from build123d import *

# Parameters (mm, degrees)
SKIZZE1_R                       = 9.5
AUFSATZ_LINEAR_AUSTRAGEN2_DEPTH = 12
SKIZZE9_R                       = 11
SCHNITT_LINEAR_AUSTRAGEN2_DEPTH = 10


with BuildPart() as part:
    # Skizze1 → Aufsatz-Linear austragen2 (new body)
    with BuildSketch(Plane.XY):
        Polygon((15, 15), (-15, 15), (-15, -40), (-5, -40), (-5, -20), (15, -20), align=None)
        Circle(SKIZZE1_R, mode=Mode.SUBTRACT)
    extrude(amount=AUFSATZ_LINEAR_AUSTRAGEN2_DEPTH)

    # Skizze9 → Schnitt-Linear austragen2 (cut)
    with BuildSketch(Plane(origin=(0, 0, 0), x_dir=(-1, 0, 0), z_dir=(0, 0, -1))):
        Circle(SKIZZE9_R)
    extrude(amount=-SCHNITT_LINEAR_AUSTRAGEN2_DEPTH, mode=Mode.SUBTRACT)


solid = part.part
Could you check a few things on this model? Use its own coordinates, in mm. A direction names the side the tool comes from. Give positions to 0.01 mm unless a question says otherwise; leave off trailing zeros. Write each loop counter-clockwise with the first axis right and the second up, starting at its lowest first coordinate (ties: lowest second). Pieces come first, ordered by that corner, then holes. Notation, with made-up numbers: (76.25, 13.5) - (102.25, 13.5) arc R24 ccw to (102.25, 27.5) - close; hole circle Ø3 at (62, 24.5). An arc over 180 degrees is marked (long way). Use CSV: the item, a comma, the result in double quotes. Start each with the question number.
Item 1: I want a section at B-B, the plane y = 0. Please give me the cut outline in (x, z), then the cut area to 3 significant figures.
Item 2: I'm going to push a flat-ended pin straight in: pin 1 (3.5 mm diameter, centred on x = 9.5, z = 8.5, fed in from -Y). Where does the tip first touch, or does it pass through?
Item 3: If I drill on line 1 along X through (y, z) = (0, 11.1); line 2 along Y through (x, z) = (0, 10.6); line 3 along X through (y, z) = (-25, 11.75), over which ranges is the centre line in solid material (lowest first)?
Item 4: I want a section at C-C, the plane z = 2.75. Please give me the cut outline in (x, y).
Item 5: For faces 4 (the face through (-10, -40, 6)), 5 (the face through (2.38, -10.74, 4.93)), 6 (the face through (-5, -30, 6)), which set-ups out of +Z, -Z, +X, -X, +Y, -Y let a thin tool reach every point of the face, with its end or its side?
Item 6: If we mould it in two halves opening along Y, with no side actions, what happens to faces 1 (the face through (0, 15, 6)), 2 (the face through (5, -20, 6)), 3 (the face through (4.38, -8.43, 10.99))? For each: pulls with the +Y half, pulls with the -Y half, needs draft (parallel to the pull), parting line crosses it, or undercut.
Item 7: I want a section at D-D, the plane y = -29. Please give me the cut outline in (x, z), then the cut area to 3 significant figures.
Item 8: I want a section at A-A, the plane x = 0. Please give me the cut outline in (y, z), then the cut area to 3 significant figures.
Findings:
1,outline,"(-15, 0) - (-11, 0) - (-11, 10) - (-9.5, 10) - (-9.5, 12) - (-15, 12) - close; (9.5, 10) - (11, 10) - (11, 0) - (15, 0) - (15, 12) - (9.5, 12) - close"
1,area,"102 mm2"
2,pin 1,"stops at y = -20"
3,line 1,"x = -15 to -9.5, 9.5 to 15"
3,line 2,"y = -20 to -9.5, 9.5 to 15"
3,line 3,"x = -15 to -5"
4,outline,"(-15, -40) - (-5, -40) - (-5, -20) - (15, -20) - (15, 15) - (-15, 15) - close; hole circle Ø22 at (0, 0)"
5,face 4,"+Z, -Z, +X, -X, -Y"
5,face 5,"-Z"
5,face 6,"+Z, -Z, +X, -Y"
6,face 1,"pulls with the +Y half"
6,face 2,"pulls with the -Y half"
6,face 3,"undercut"
7,outline,"(-15, 0) - (-5, 0) - (-5, 12) - (-15, 12) - close"
7,area,"120 mm2"
8,outline,"(-20, 0) - (-11, 0) - (-11, 10) - (-9.5, 10) - (-9.5, 12) - (-20, 12) - close; (9.5, 10) - (11, 10) - (11, 0) - (15, 0) - (15, 12) - (9.5, 12) - close"
8,area,"162 mm2"
